The figure shows three views and two pictorial views of one solid part (mm, origin at its lowest corner). Answer the questions. A direction names the side the tool comes from. Round coordinates to 2 decimals unless told otherwise and drop trailing zeros. Write each loop counter-clockwise with the first axis right and the second up, starting at its lowest first coordinate (ties: lowest second). Pieces come first, ordered by that corner, then holes.
Item 1: Find section A-A on y = 13.75. Give the vertices of the cut face in (x, z), then the cut area to 3 significant figures.
Item 2: A tool of negligible diameter and unlimited length cuts with its end or side. For the marked faces 1, 2 and 3, from which of +Z, -Z, +X, -X, +Y, -Y can it reach the whole face along a straight path? Write none if from no direction.
Item 3: Find the intervals of material crossed by probe 1 along Z at (x, y) = (10.5, 15.5); probe 2 along Z at (x, y) = (16, 9); probe 3 along Y at (x, z) = (13.75, 5), in increasing order.
Item 4: Each of these flat-tipped pins is pushed along its axis until it touches: pin 1 (1 mm diameter, centred on x = 24, z = 14, fed in from +Y) (1 decimal); pin 2 (10 mm diameter, centred on y = 23, z = 26.5, fed in from -X); pin 3 (2 mm diameter, centred on x = 13.5, y = 21.5, fed in from +Z); pin 4 (14 mm diameter, centred on x = 10.5, y = 20, fed in from -Z). Where does it stop, or does it pass through?
Item 5: Find section C-C on z = 21.5. Give the vertices of the cut face in (x, y), then the cut area to 3 significant figures.
Item 6: Find section D-D on y = 8. Give the vertices of the cut face in (x, z).
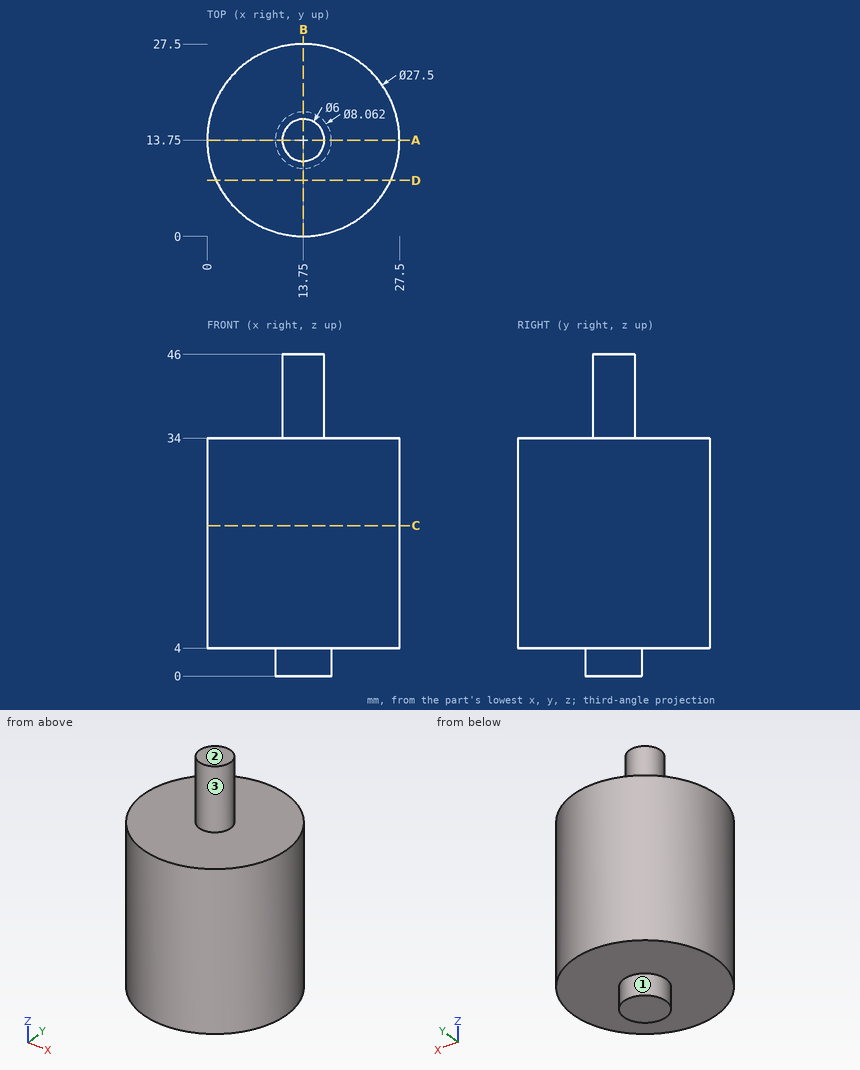
Check values:
1. outline: (0, 4) - (9.72, 4) - (9.72, 0) - (17.78, 0) - (17.78, 4) - (27.5, 4) - (27.5, 34) - (16.75, 34) - (16.75, 46) - (10.75, 46) - (10.75, 34) - (0, 34) - close
1. area: 929 mm2
2. face 1: -Z
2. face 2: +Z, +X, -X, +Y, -Y
2. face 3: +Z
3. probe 1: z = 0 to 34
3. probe 2: z = 4 to 34
3. probe 3: y = 0 to 27.5
4. pin 1: stops at y = 23.4
4. pin 2: stops at x = 0.67
4. pin 3: stops at z = 34
4. pin 4: stops at z = 0
5. outline: circle Ø27.5 at (13.75, 13.75)
5. area: 594 mm2
6. outline: (1.26, 4) - (26.24, 4) - (26.24, 34) - (1.26, 34) - close
